```python
from build123d import *

# Parameters (mm, degrees)
F1_DEPTH = 9
F2_W     = 9
F2_H     = 5
F3_DEPTH = 3
F5_DEPTH = 25


with BuildPart() as f1:
    # F0 (on Front) → F1 (new body)
    with BuildSketch(Plane.XZ):
        with BuildLine():
            Line((-48.888732, 31.176301), (-48.888732, 37.676301))
            ThreePointArc((-48.888732, 37.676301), (-56.388732, 30.176301), (-48.888732, 22.676301))
            Line((-48.888732, 22.676301), (-48.888732, 29.176301))
            ThreePointArc((-48.888732, 29.176301), (-49.888732, 30.176301), (-48.888732, 31.176301))
        make_face()
        with BuildLine():
            ThreePointArc((-48.888732, 22.676301), (-43.585431, 24.873), (-41.388732, 30.176301))
            ThreePointArc((-41.388732, 30.176301), (-43.585431, 35.479602), (-48.888732, 37.676301))
            Line((-48.888732, 37.676301), (-48.888732, 31.176301))
            ThreePointArc((-48.888732, 31.176301), (-48.181625, 30.883408), (-47.888732, 30.176301))
            ThreePointArc((-47.888732, 30.176301), (-48.181625, 29.469194), (-48.888732, 29.176301))
            Line((-48.888732, 29.176301), (-48.888732, 22.676301))
        make_face()
        with BuildLine():
            ThreePointArc((-48.888732, 37.676301), (-43.585431, 35.479602), (-41.388732, 30.176301))
            Line((-41.388732, 30.176301), (-41.388732, 37.676301))
            Line((-41.388732, 37.676301), (-48.888732, 37.676301))
        make_face()
        with BuildLine():
            Line((-41.388732, 22.676301), (-41.388732, 30.176301))
            ThreePointArc((-41.388732, 30.176301), (-43.585431, 24.873), (-48.888732, 22.676301))
            Line((-48.888732, 22.676301), (-41.388732, 22.676301))
        make_face()
    extrude(amount=F1_DEPTH)

    # F2 (on face) → F3 (join)
    with BuildSketch(Plane.YZ.offset(-41.388732)):
        with Locations((-4.5, 35.176301)):
            Rectangle(F2_W, F2_H)
        with Locations((-4.5, 25.176301)):
            Rectangle(F2_W, F2_H)
    extrude(amount=F3_DEPTH)

    # F4 (on face) → F5 (cut)
    with BuildSketch(Plane.YZ.offset(-38.388732)):
        with BuildLine():
            Line((5.874889, 26.795391), (2.194733, 26.795391))
            ThreePointArc((2.194733, 26.795391), (-4.5, 22.676301), (-11.194733, 26.795391))
            Line((-11.194733, 26.795391), (-12.804028, 26.795391))
            Line((-12.804028, 26.795391), (-12.804028, 21.1592))
            Line((-12.804028, 21.1592), (5.874889, 21.1592))
            Line((5.874889, 21.1592), (5.874889, 26.795391))
        make_face()
        with BuildLine():
            ThreePointArc((-4.5, 37.676301), (-2.128292, 37.291426), (0, 36.176301))
            Line((0, 36.176301), (0, 37.676301))
            Line((0, 37.676301), (-4.5, 37.676301))
        make_face()
        with BuildLine():
            ThreePointArc((-9, 36.176301), (-6.871708, 37.291426), (-4.5, 37.676301))
            Line((-4.5, 37.676301), (-9, 37.676301))
            Line((-9, 37.676301), (-9, 36.176301))
        make_face()
    extrude(amount=-F5_DEPTH, mode=Mode.SUBTRACT)


solid = f1.part
```
CAD build for the part. Positions are in the model's coordinates, mm. A direction names the side the tool comes from. Coordinates: 2 decimals unless noted, no trailing zeros. Write each loop counter-clockwise with the first axis right and the second up, starting at its lowest first coordinate (ties: lowest second). Pieces come first, ordered by that corner, then holes. Notation, with made-up numbers: (-32.75, 78.5) -> (9.25, 78.5) arc R8 ccw to (9.25, 82.5) -> close; hole circle Ø3 at (56, 42). An arc over 180 degrees is marked (long way). Return JSON: item names as keys, results as strings. Group by question number.
Q1. Pull direction Z, two halves, no side cores. Call faces 3 (the face through (-40, -5, 27.676)), 4 (the face through (-40, -5, 32.676)), 5 (the face through (-47.5, -9, 30.1)), 6 (the face through (-56.387, -4.437, 30.341)): released by +Z, released by -Z, zero draft, split by the parting line, or undercut.
Q2. Drill centre lines: line 1 (X direction, y = -5.75, z = 30); line 2 (Z direction, x = -39.25, y = -6.25); line 3 (Z direction, x = -39.5, y = -3.5). Where is each one in solid material? Low to high.
Q3. Which spindle directions (+Z, -Z, +X, -X, +Y, -Y) get a long thin tool onto all of the face, cutting with end or side? Do faces 1 (the face through (-44.117, -4.432, 22.677)), 2 (the face through (-41.389, -4, 30)). Say none if no direction does.
Q4. Cut at C-C, the plane x = -50.5. Give the cut face in (y, z), then the cut area to 3 significant figures.
Q5. Cut at A-A, the plane x = -41. Give the cut face in (y, z).
Q6. Flat gauge pins, fed straight in: pin 1 (1.5 mm diameter, centred on y = -4.5, z = 31, fed in from +X); pin 2 (1.5 mm diameter, centred on x = -40, y = -3.5, fed in from +Z). Where does each tip first touch, or does it go through?
Q7. Cut at B-B, the plane y = -1.75. Give the cut face in (x, z).
Q8. Cut at D-D, the plane y = -3. Give the cut face in (x, z).
Returned:
{
 "1": {"face 3": "undercut", "face 4": "undercut", "face 5": "zero draft", "face 6": "split by the parting line"},
 "2": {"line 1": "x = -56.39 to -49.87, -47.9 to -41.39", "line 2": "z = 22.88 to 27.68, 32.68 to 37.47", "line 3": "z = 22.74 to 27.68, 32.68 to 37.61"},
 "3": {"face 1": "-Z, +X, -X", "face 2": "+X, +Y, -Y"},
 "4": {"outline": "(-9, 24.18) arc R7.5 ccw to (-6.11, 22.85) -> (-2.89, 22.85) arc R7.5 ccw to (0, 24.18) -> (0, 36.18) arc R7.5 ccw to (-2.89, 37.5) -> (-6.11, 37.5) arc R7.5 ccw to (-9, 36.18) -> close", "area": "126 mm2"},
 "5": {"outline": "(-9, 24.18) arc R7.5 ccw to (0, 24.18) -> (0, 27.68) -> (-9, 27.68) -> close; (-9, 32.68) -> (0, 32.68) -> (0, 36.18) arc R7.5 ccw to (-4.5, 37.68) arc R7.5 ccw to (-9, 36.18) -> close"},
 "6": {"pin 1": "stops at x = -41.39", "pin 2": "stops at z = 37.67"},
 "7": {"outline": "(-51.64, 23.2) -> (-38.39, 23.2) -> (-38.39, 27.68) -> (-41.39, 27.68) -> (-41.39, 32.68) -> (-38.39, 32.68) -> (-38.39, 37.15) -> (-51.64, 37.15) arc R7.5 ccw to start; hole (-48.89, 29.18) arc R1 ccw to (-47.89, 30.18) arc R1 ccw (long way) to start"},
 "8": {"outline": "(-50.39, 22.83) -> (-38.39, 22.83) -> (-38.39, 27.68) -> (-41.39, 27.68) -> (-41.39, 32.68) -> (-38.39, 32.68) -> (-38.39, 37.52) -> (-50.39, 37.52) arc R7.5 ccw to start; hole (-48.89, 29.18) arc R1 ccw to (-47.89, 30.18) arc R1 ccw (long way) to start"}
}
